Build history of the part. All positions in model axes, mm. A direction names the side the tool comes from. Give positions to 0.01 mm unless a question says otherwise; leave off trailing zeros. Order: outer loops, then holes, each group sorted by start corner. A loop starts at its lowest first (then second) coordinate and runs counter-clockwise, first axis right, second up. Notation, with made-up numbers: (8.25, 71) -> (67.25, 71) arc R18 cw to (67.25, 92) -> close; hole circle Ø6 at (-23.5, 78.25). An arc over 180 degrees is marked (long way). One line per question, with ' | ' between items. Start each with the question number.
(1) Which spindle directions (+Z, -Z, +X, -X, +Y, -Y) get a long thin tool onto all of the face, cutting with end or side? Do faces 5 (the face through (0.76, 35.49, -55.31)), 6 (the face through (0.76, 35.49, 55.31)). Say none if no direction does.
(2) Cut at C-C (z = 26). Give the cut face in (x, y), then the cut area to 3 significant figures.
(3) Cut at B-B (x = -10.5). Give the cut face in (y, z).
(4) Cut at A-A (y = 0). Give the cut face in (x, z).
(5) Pin check, flat tips, straight feed: pin 1 Ø5 at (x, z) = (-21.5, -38) entering from -Y; pin 2 Ø5 at (x, z) = (8.5, 44) entering from -Y; pin 3 Ø4 at (y, z) = (11, 24) entering from +X; pin 4 Ø10 at (x, y) = (-18, -12.5) entering from +Z. Stop position of each tip, or through.
(6) Drill centre lines: L1, parallel to X at y = -17.25, z = -53.5; L2, parallel to X at y = -0.5, z = 22; L3, parallel to X at y = 17, z = -43. Where is each one in solid material? Low to high. Write a range as from..to.
(7) Pull direction Y, two halves, no side cores. Call faces 1 (the face through (29.5, -18.44, 55.31)), 2 (the face through (17.535, -33.713, 0.833)), 3 (the face through (31, 16.7, 55.3)), 4 (the face through (-2.99, 31.14, -59.5)): +Y half, -Y half, draft (parallel to the pull), parting line (faces both ways), or undercut.
from build123d import *

# Parameters (mm, degrees)
SKETCH_1_R                  = 38
SKETCH_1_R_2                = 31.1
EXTRUDE_1_DEPTH             = 59.5
HOLE_WIZARD_M3_1_AT_2_COUNT = 2
HOLE_WIZARD_M3_1_AT_2_PITCH = 34.5
HOLE_WIZARD_M3_1_AT_3_COUNT = 2
HOLE_WIZARD_M3_1_AT_3_PITCH = 59.755752861
HOLE_WIZARD_M3_1_AT_4_COUNT = 2
HOLE_WIZARD_M3_1_AT_4_PITCH = 69
HOLE_WIZARD_M3_1_AT_5_COUNT = 2
HOLE_WIZARD_M3_1_AT_5_PITCH = 59.755752861
HOLE_WIZARD_M3_1_AT_6_COUNT = 2
HOLE_WIZARD_M3_1_AT_6_PITCH = 34.5


with BuildPart() as part:
    # 草图1 → 凸台-拉伸1 (new, symmetric)
    with BuildSketch(Plane.XY):
        Circle(SKETCH_1_R)
        Circle(SKETCH_1_R_2, mode=Mode.SUBTRACT)
    extrude(amount=EXTRUDE_1_DEPTH, both=True)

    # 草图2 → M3 螺纹孔1 (revolve, cut)
    with BuildSketch(Plane(origin=(0, 34.5, 59.5), x_dir=(0, -1, 0), z_dir=(1, 0, 0))):
        Polygon((0, 0), (0, 9.251075774), (1.25, 8.5), (1.25, 0), align=None)
    hole_wizard_m3_1 = revolve(axis=Axis((0, 34.5, 65.85), (0, 0, -1)), mode=Mode.SUBTRACT)

    # M3 螺纹孔1 at 2: M3 螺纹孔1 ×2
    with Locations(*[Vector(0.8660254037844671, -0.49999999999995076, 0) * (i * HOLE_WIZARD_M3_1_AT_2_PITCH) for i in range(1, HOLE_WIZARD_M3_1_AT_2_COUNT)]):
        add(hole_wizard_m3_1, mode=Mode.SUBTRACT)

    # M3 螺纹孔1 at 3: M3 螺纹孔1 ×2
    with Locations(*[Vector(0.5000000000000492, -0.8660254037844103, 0) * (i * HOLE_WIZARD_M3_1_AT_3_PITCH) for i in range(1, HOLE_WIZARD_M3_1_AT_3_COUNT)]):
        add(hole_wizard_m3_1, mode=Mode.SUBTRACT)

    # M3 螺纹孔1 at 4: M3 螺纹孔1 ×2
    with Locations(*[(0, -i * HOLE_WIZARD_M3_1_AT_4_PITCH, 0) for i in range(1, HOLE_WIZARD_M3_1_AT_4_COUNT)]):
        add(hole_wizard_m3_1, mode=Mode.SUBTRACT)

    # M3 螺纹孔1 at 5: M3 螺纹孔1 ×2
    with Locations(*[Vector(-0.49999999999995076, -0.866025403784467, 0) * (i * HOLE_WIZARD_M3_1_AT_5_PITCH) for i in range(1, HOLE_WIZARD_M3_1_AT_5_COUNT)]):
        add(hole_wizard_m3_1, mode=Mode.SUBTRACT)

    # M3 螺纹孔1 at 6: M3 螺纹孔1 ×2
    with Locations(*[Vector(-0.8660254037844105, -0.5000000000000487, 0) * (i * HOLE_WIZARD_M3_1_AT_6_PITCH) for i in range(1, HOLE_WIZARD_M3_1_AT_6_COUNT)]):
        add(hole_wizard_m3_1, mode=Mode.SUBTRACT)

    # 镜向1: M3 螺纹孔1 across plane
    add(hole_wizard_m3_1.mirror(Plane.XY), mode=Mode.SUBTRACT)

    # 镜向1 copy 1 sketch → 镜向1 copy 1 (revolve, cut)
    with BuildSketch(Plane(origin=(29.877876431, 17.25, -59.5), x_dir=(0, -1, 0), z_dir=(1, 0, 0))):
        Polygon((0, 0), (0, -9.251075774), (1.25, -8.5), (1.25, 0), align=None)
    revolve(axis=Axis((29.877876431, 17.25, -65.85), (0, 0, -1)), mode=Mode.SUBTRACT)

    # 镜向1 copy 2 sketch → 镜向1 copy 2 (revolve, cut)
    with BuildSketch(Plane(origin=(29.877876431, -17.25, -59.5), x_dir=(0, -1, 0), z_dir=(1, 0, 0))):
        Polygon((0, 0), (0, -9.251075774), (1.25, -8.5), (1.25, 0), align=None)
    revolve(axis=Axis((29.877876431, -17.25, -65.85), (0, 0, -1)), mode=Mode.SUBTRACT)

    # 镜向1 copy 3 sketch → 镜向1 copy 3 (revolve, cut)
    with BuildSketch(Plane(origin=(0, -34.5, -59.5), x_dir=(0, -1, 0), z_dir=(1, 0, 0))):
        Polygon((0, 0), (0, -9.251075774), (1.25, -8.5), (1.25, 0), align=None)
    revolve(axis=Axis((0, -34.5, -65.85), (0, 0, -1)), mode=Mode.SUBTRACT)

    # 镜向1 copy 4 sketch → 镜向1 copy 4 (revolve, cut)
    with BuildSketch(Plane(origin=(-29.877876431, -17.25, -59.5), x_dir=(0, -1, 0), z_dir=(1, 0, 0))):
        Polygon((0, 0), (0, -9.251075774), (1.25, -8.5), (1.25, 0), align=None)
    revolve(axis=Axis((-29.877876431, -17.25, -65.85), (0, 0, -1)), mode=Mode.SUBTRACT)

    # 镜向1 copy 5 sketch → 镜向1 copy 5 (revolve, cut)
    with BuildSketch(Plane(origin=(-29.877876431, 17.25, -59.5), x_dir=(0, -1, 0), z_dir=(1, 0, 0))):
        Polygon((0, 0), (0, -9.251075774), (1.25, -8.5), (1.25, 0), align=None)
    revolve(axis=Axis((-29.877876431, 17.25, -65.85), (0, 0, -1)), mode=Mode.SUBTRACT)


solid = part.part
Result set:
1) face 5: -Z | face 6: +Z
2) outline: circle Ø76 at (0, 0); hole circle Ø62.2 at (0, 0) | area: 1,500 mm2
3) outline: (-36.52, -59.5) -> (-29.27, -59.5) -> (-29.27, 59.5) -> (-36.52, 59.5) -> close; (29.27, -59.5) -> (36.52, -59.5) -> (36.52, 59.5) -> (29.27, 59.5) -> close
4) outline: (-38, -59.5) -> (-31.1, -59.5) -> (-31.1, 59.5) -> (-38, 59.5) -> close; (31.1, -59.5) -> (38, -59.5) -> (38, 59.5) -> (31.1, 59.5) -> close
5) pin 1: stops at y = -32.91 | pin 2: stops at y = -37.52 | pin 3: stops at x = 36.92 | pin 4: passes through
6) L1: x = -33.86..-31.13, -28.63..-25.88, 25.88..28.63, 31.13..33.86 | L2: x = -38..-31.1, 31.1..38 | L3: x = -33.99..-26.04, 26.04..33.99
7) face 1: undercut | face 2: parting line | face 3: undercut | face 4: draft
